from build123d import *

# Parameters (mm, degrees)
SKETCH1_R           = 37.5
SKETCH1_R_2         = 29.5
BOSS_EXTRUDE1_DEPTH = 11
SKETCH2_R           = 1
CUT_EXTRUDE1_DEPTH  = 11
SKETCH3_R           = 32.5
CUT_EXTRUDE2_DEPTH  = 4


with BuildPart() as part:
    # Sketch1 → Boss-Extrude1 (new body)
    with BuildSketch(Plane.XY):
        Circle(SKETCH1_R)
        Circle(SKETCH1_R_2, mode=Mode.SUBTRACT)
    extrude(amount=BOSS_EXTRUDE1_DEPTH)

    # Sketch2 → Cut-Extrude1 (cut)
    with BuildSketch(Plane(origin=(0, 0, 0), x_dir=(-1, 0, 0), z_dir=(0, 0, -1))):
        with Locations((-17, 29.444863729)):
            Circle(SKETCH2_R)
        with Locations((17, 29.444863729)):
            Circle(SKETCH2_R)
        with Locations((34, 0)):
            Circle(SKETCH2_R)
        with Locations((17, -29.444863729)):
            Circle(SKETCH2_R)
        with Locations((-17, -29.444863729)):
            Circle(SKETCH2_R)
        with Locations((-34, 0)):
            Circle(SKETCH2_R)
    extrude(amount=-CUT_EXTRUDE1_DEPTH, mode=Mode.SUBTRACT)

    # Sketch3 → Cut-Extrude2 (cut)
    with BuildSketch(Plane.XY.offset(11)):
        Circle(SKETCH3_R)
    extrude(amount=-CUT_EXTRUDE2_DEPTH, mode=Mode.SUBTRACT)


solid = part.part
Design review of the part built by this model. Coordinates are the model's own, in mm. A direction names the side the tool comes from. Give positions to 0.01 mm unless a question says otherwise; leave off trailing zeros. Loops run counter-clockwise (first coordinate to the right, second up) from the corner with the lowest first, then second, coordinate; pieces in that order, holes last. Notation, with made-up numbers: (41, 88.5) - (70, 88.5) arc R30 cw to (70, 113.5) - close; hole circle Ø9 at (43.25, 50.5). An arc over 180 degrees is marked (long way). Write item = value, one per line.
1) Take a section at B-B on x = 0. State the section outline as (y, z) points, and give its area (3 significant figures).
Result sheet:
outline = (-37.5, 0) - (-29.5, 0) - (-29.5, 7) - (-32.5, 7) - (-32.5, 11) - (-37.5, 11) - close; (29.5, 0) - (37.5, 0) - (37.5, 11) - (32.5, 11) - (32.5, 7) - (29.5, 7) - close
area = 152 mm2
2) Take a section at A-A on y = 0. State the section outline as (x, z) points.
Result sheet:
outline = (-37.5, 0) - (-35, 0) - (-35, 11) - (-37.5, 11) - close; (-33, 0) - (-29.5, 0) - (-29.5, 7) - (-32.5, 7) - (-32.5, 11) - (-33, 11) - close; (29.5, 0) - (33, 0) - (33, 11) - (32.5, 11) - (32.5, 7) - (29.5, 7) - close; (35, 0) - (37.5, 0) - (37.5, 11) - (35, 11) - close
3) Clearance check with flat-ended pins moving along their axes: pin 1 Ø1 at (x, z) = (-29.5, 8.5) entering from -Y (3 decimals); pin 2 Ø6 at (y, z) = (-27, 7.5) entering from +X; pin 3 Ø1 at (y, z) = (8, 2.5) entering from +X; pin 4 Ø2.5 at (x, y) = (-34, 0) entering from +Z. State where each tip first meets the part, or that it passes through.
Result sheet:
pin_1 = -23.775
pin_2 = 28.81
pin_3 = 36.74
pin_4 = 11
4) Draft analysis for pull direction Y (two halves, no side actions). For faces 3 (the face through (-35, 0, 5)), 4 (the face through (-11, -28, 0)), 5 (the face through (-4.88, 37.18, 5.42)), state which applies: +Y half, -Y half, draft (parallel to the pull), parting line (faces both ways), or undercut.
Result sheet:
face_3 = undercut
face_4 = draft
face_5 = parting line
5) To check wall thickness, follow line 1 (X direction, y = 29.5, z = 7.75); line 2 (Y direction, x = -17, z = 2.5); line 3 (Z direction, x = 29, y = -7.5). State the ranges of each line that lie inside material, in increasing order.
Result sheet:
line_1 = -23.15 to -18, -16 to -13.64, 13.64 to 16, 18 to 23.15
line_2 = -33.43 to -30.44, -28.44 to -24.11, 24.11 to 28.44, 30.44 to 33.43
line_3 = 0 to 7
6) Take a section at C-C on y = -18. State the section outline as (x, z) points, and give its area (3 significant figures).
Result sheet:
outline = (-32.9, 0) - (-23.37, 0) - (-23.37, 7) - (-27.06, 7) - (-27.06, 11) - (-32.9, 11) - close; (23.37, 0) - (32.9, 0) - (32.9, 11) - (27.06, 11) - (27.06, 7) - (23.37, 7) - close
area = 180 mm2
7) Take a section at D-D on z = 3.75. State the section outline as (x, y) points.
Result sheet:
outline = circle Ø75 at (0, 0); hole circle Ø2 at (-34, 0); hole circle Ø59 at (0, 0); hole circle Ø2 at (-17, -29.44); hole circle Ø2 at (-17, 29.44); hole circle Ø2 at (17, -29.44); hole circle Ø2 at (17, 29.44); hole circle Ø2 at (34, 0)
8) Tool access review of faces 1 (the face through (31, 9.76, 9.03)), 2 (the face through (-28, 17, 11)): name each direction out of +Z, -Z, +X, -X, +Y, -Y from which nothing blocks a thin tool from reaching the whole face with its end or side.
Result sheet:
face_1 = +Z
face_2 = +Z, +X, -X, +Y, -Y
